For this review, take the finished solid that the model builds, in its own axes (mm). Face numbers are marked on the shaded views. A direction names the side the tool comes from. Give positions to 0.01 mm unless a question says otherwise; leave off trailing zeros. Loops run counter-clockwise (first coordinate to the right, second up) from the corner with the lowest first, then second, coordinate; pieces in that order, holes last. Notation, with made-up numbers: (40, 2) -> (48, 2) arc R25 ccw to (48, 24) -> close; hole circle Ø6 at (-16.75, 46.5). An arc over 180 degrees is marked (long way). Answer as CSV lines item,"result". Start each with the question number.
Item 1: Add section B-B on z = 0. State the section outline as (x, y) points.
Item 2: The part is to be moulded in two halves that separate along Z. For the marked faces 1, 2 and 3, say which applies: +Z half, -Z half, draft (parallel to the pull), parting line (faces both ways), or undercut.
Item 3: For L1, parallel to Z at x = 0, y = 2; L2, parallel to X at y = 9.3, z = 0; L3, parallel to Z at x = 9.5, y = 10.25, list the stretches that pass through material, from the lowest coordinate up. Write a range as from..to.
Item 4: Add section C-C on y = 11.5. State how many separate pieces and enclosed holes the cut face has, plus the area to 3 significant figures.
Item 5: Add section A-A on x = 0. State the section outline as (y, z) points, plus the area to 3 significant figures.
Item 6: Clearance check with flat-ended pins moving along their axes: P1, Ø4, axis at y = 5, z = -6, coming from the -X side; P2, Ø1.5, axis at x = -0.5, z = 39.5, coming from the +Y side; P3, Ø5, axis at x = -11.5, y = 9, coming from the -Z side; P4, Ø2, axis at x = -33, z = -19.05, coming from the -Y side. State where each tip first meets the part, or that it passes through.
Item 7: Machinability: for the marked faces 4 and 5, which of the approach directions +Z, -Z, +X, -X, +Y, -Y give a long, thin tool a straight path to every point of the face, cutting with its end or side? Answer none if there is none.
Item 8: Add section D-D on z = 19.05. State the section outline as (x, y) points, plus the area to 3 significant figures.
```python
from build123d import *

# Parameters (mm, degrees)
SKETCH1_R                                        = 45.466
BOSS_EXTRUDE1_DEPTH                              = 25.4
SKETCH3_R                                        = 20.32
CUT_EXTRUDE1_DEPTH                               = 12.7
CSK_FOR_1_4_FLAT_HEAD_MACHINE_SCREW1_D           = 6.5278
CSK_FOR_1_4_FLAT_HEAD_MACHINE_SCREW1_DEPTH       = 25.4
CSK_FOR_1_4_FLAT_HEAD_MACHINE_SCREW1_CSINK_D     = 12.8778
CSK_FOR_1_4_FLAT_HEAD_MACHINE_SCREW1_CSINK_ANGLE = 82
CSK_FOR_1_4_FLAT_HEAD_MACHINE_SCREW1_TIP         = 1.961148974
SKETCH8_R                                        = 46.955588052
CUT_EXTRUDE2_DEPTH                               = 12.7
SKETCH4_R                                        = 1.778
CUT_EXTRUDE3_DEPTH                               = 13.7
SKETCH9_R                                        = 2.54
CUT_EXTRUDE4_DEPTH                               = 5.08
CIRPATTERN1_COUNT                                = 24
SKETCH10_R                                       = 22.834776664
BOSS_EXTRUDE2_DEPTH                              = 5.08
SKETCH11_R                                       = 3.302
CUT_EXTRUDE5_DEPTH                               = 13.7


with BuildPart() as part:
    # Sketch1 → Boss-Extrude1 (new body)
    with BuildSketch(Plane(origin=(0, 0, 0), x_dir=(1, 0, 0), z_dir=(0, 1, 0))):
        Circle(SKETCH1_R)
    extrude(amount=BOSS_EXTRUDE1_DEPTH)

    # Sketch3 → Cut-Extrude1 (cut)
    with BuildSketch(Plane.XZ):
        Circle(SKETCH3_R)
    extrude(amount=-CUT_EXTRUDE1_DEPTH, mode=Mode.SUBTRACT)

    # CSK for 1/4 Flat Head Machine Screw1
    with Locations(Plane(origin=(0, 25.4, 0), x_dir=(1, 0, 0), z_dir=(0, 1, 0))):
        with Locations((0, 0)):
            CounterSinkHole(CSK_FOR_1_4_FLAT_HEAD_MACHINE_SCREW1_D / 2, CSK_FOR_1_4_FLAT_HEAD_MACHINE_SCREW1_CSINK_D / 2, depth=CSK_FOR_1_4_FLAT_HEAD_MACHINE_SCREW1_DEPTH, counter_sink_angle=CSK_FOR_1_4_FLAT_HEAD_MACHINE_SCREW1_CSINK_ANGLE)
            with Locations((0, 0, -(CSK_FOR_1_4_FLAT_HEAD_MACHINE_SCREW1_DEPTH + CSK_FOR_1_4_FLAT_HEAD_MACHINE_SCREW1_TIP / 2))):  # 118° drill point
                Cone(0, CSK_FOR_1_4_FLAT_HEAD_MACHINE_SCREW1_D / 2, CSK_FOR_1_4_FLAT_HEAD_MACHINE_SCREW1_TIP, mode=Mode.SUBTRACT)

    # Sketch8 → Cut-Extrude2 (cut)
    with BuildSketch(Plane(origin=(0, 25.4, 0), x_dir=(1, 0, 0), z_dir=(0, 1, 0))):
        Circle(SKETCH8_R)
    extrude(amount=-CUT_EXTRUDE2_DEPTH, mode=Mode.SUBTRACT)

    # Sketch4 → Cut-Extrude3 (cut, through all)
    with BuildSketch(Plane.XZ):
        with Locations((0, 38.1)):
            Circle(SKETCH4_R)
    cut_extrude3 = extrude(amount=-CUT_EXTRUDE3_DEPTH, mode=Mode.SUBTRACT)

    # Sketch9 → Cut-Extrude4 (cut)
    with BuildSketch(Plane(origin=(0, 12.7, 0), x_dir=(1, 0, 0), z_dir=(0, 1, 0))):
        with Locations((0, -38.1)):
            Circle(SKETCH9_R)
    cut_extrude4 = extrude(amount=-CUT_EXTRUDE4_DEPTH, mode=Mode.SUBTRACT)

    # CirPattern1: Cut-Extrude3, Cut-Extrude4 ×24 about axis
    cirpattern1_axis = Axis((0, 0, 0), (0, 1, 0))
    for i in range(1, CIRPATTERN1_COUNT):
        add(cut_extrude3.rotate(cirpattern1_axis, i * 360 / CIRPATTERN1_COUNT), mode=Mode.SUBTRACT)
        add(cut_extrude4.rotate(cirpattern1_axis, i * 360 / CIRPATTERN1_COUNT), mode=Mode.SUBTRACT)

    # Sketch10 → Boss-Extrude2 (add)
    with BuildSketch(Plane(origin=(0, 12.7, 0), x_dir=(1, 0, 0), z_dir=(0, 1, 0))):
        Circle(SKETCH10_R)
    extrude(amount=-BOSS_EXTRUDE2_DEPTH)

    # Sketch11 → Cut-Extrude5 (cut, through all)
    with BuildSketch(Plane(origin=(0, 12.7, 0), x_dir=(1, 0, 0), z_dir=(0, 1, 0))):
        Circle(SKETCH11_R)
    extrude(amount=-CUT_EXTRUDE5_DEPTH, mode=Mode.SUBTRACT)


solid = part.part
```
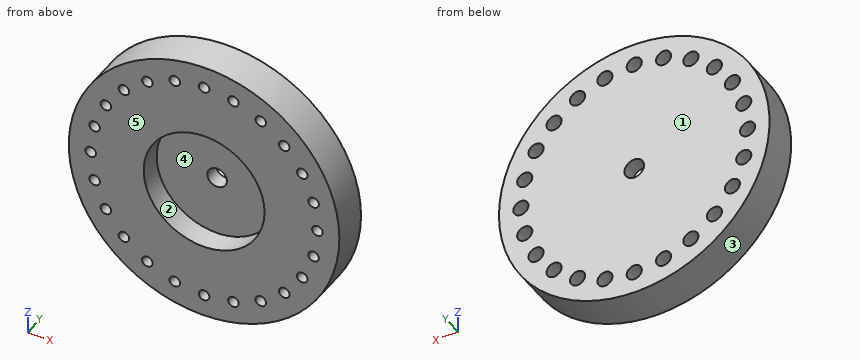
Computed values:
1,outline,"(-45.47, 0) -> (-39.88, 0) -> (-39.88, 7.62) -> (-40.64, 7.62) -> (-40.64, 12.7) -> (-45.47, 12.7) -> close; (-36.32, 0) -> (-20.32, 0) -> (-20.32, 7.62) -> (-3.3, 7.62) -> (-3.3, 12.7) -> (-35.56, 12.7) -> (-35.56, 7.62) -> (-36.32, 7.62) -> close; (3.3, 7.62) -> (20.32, 7.62) -> (20.32, 0) -> (36.32, 0) -> (36.32, 7.62) -> (35.56, 7.62) -> (35.56, 12.7) -> (3.3, 12.7) -> close; (39.88, 0) -> (45.47, 0) -> (45.47, 12.7) -> (40.64, 12.7) -> (40.64, 7.62) -> (39.88, 7.62) -> close"
2,face 1,"draft"
2,face 2,"undercut"
2,face 3,"parting line"
3,L1,"-45.47..-39.88, -36.32..-20.32, 20.32..36.32, 39.88..45.47"
3,L2,"-45.47..-40.64, -35.56..-3.3, 3.3..35.56, 40.64..45.47"
3,L3,"-44.46..-39.32, -34.29..34.29, 39.32..44.46"
4,separate pieces,"1"
4,enclosed holes,"25"
4,area,"5,970 mm²"
5,outline,"(0, -45.47) -> (12.7, -45.47) -> (12.7, -40.64) -> (7.62, -40.64) -> (7.62, -39.88) -> (0, -39.88) -> close; (0, -36.32) -> (7.62, -36.32) -> (7.62, -35.56) -> (12.7, -35.56) -> (12.7, -3.3) -> (7.62, -3.3) -> (7.62, -20.32) -> (0, -20.32) -> close; (0, 20.32) -> (7.62, 20.32) -> (7.62, 3.3) -> (12.7, 3.3) -> (12.7, 35.56) -> (7.62, 35.56) -> (7.62, 36.32) -> (0, 36.32) -> close; (0, 39.88) -> (7.62, 39.88) -> (7.62, 40.64) -> (12.7, 40.64) -> (12.7, 45.47) -> (0, 45.47) -> close"
5,area,"706 mm²"
6,P1,"x = -45.29"
6,P2,"y = 7.62"
6,P3,"z = -44.57"
6,P4,"through"
7,face 4,"-Y"
7,face 5,"+Z, -Z, +X, -X, -Y"
8,outline,"(-41.28, 0) -> (-34.77, 0) -> (-34.77, 7.62) -> (-35.54, 7.62) -> (-35.54, 12.7) -> (-41.28, 12.7) -> close; (-31.22, 0) -> (-7.07, 0) -> (-7.07, 7.62) -> (7.07, 7.62) -> (7.07, 0) -> (31.22, 0) -> (31.22, 7.62) -> (30.46, 7.62) -> (30.46, 12.7) -> (-30.46, 12.7) -> (-30.46, 7.62) -> (-31.22, 7.62) -> close; (34.77, 0) -> (41.28, 0) -> (41.28, 12.7) -> (35.54, 12.7) -> (35.54, 7.62) -> (34.77, 7.62) -> close"
8,area,"835 mm²"
